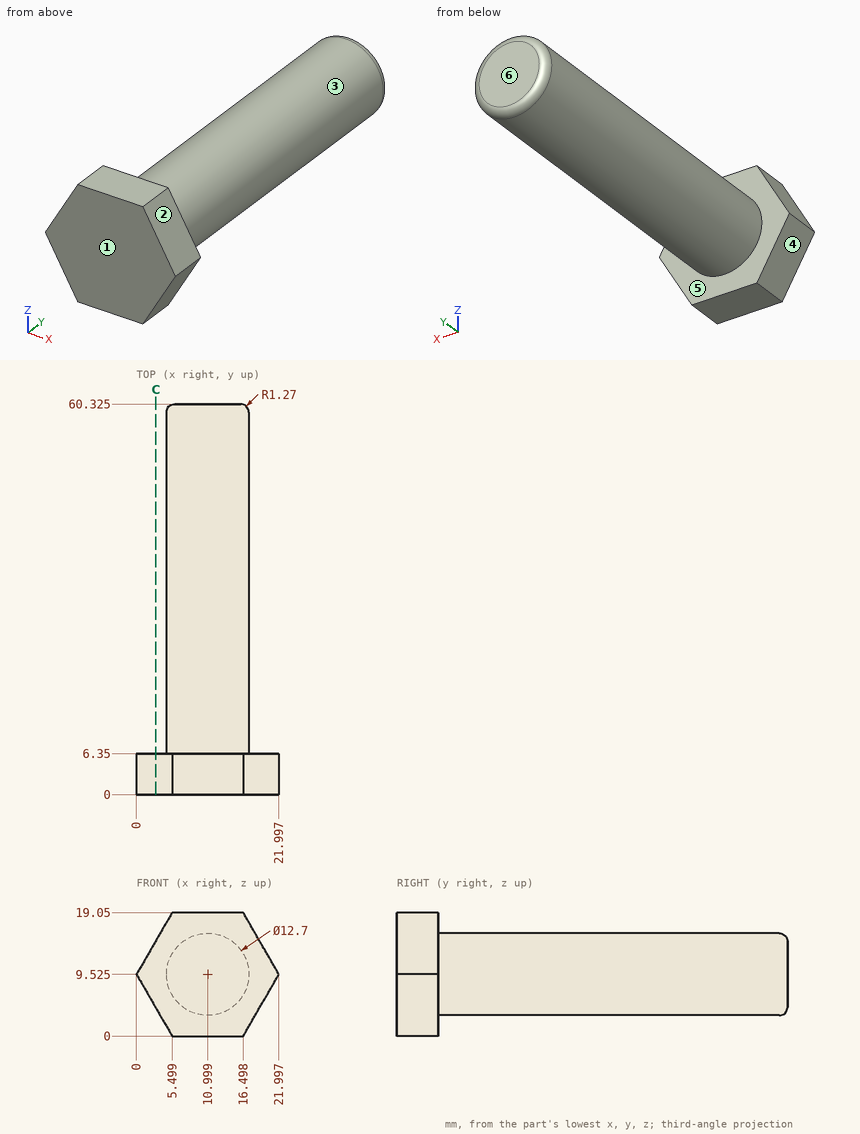
Here's the drawing with two shaded views (mm, measured from the low corner). I have some questions. A direction names the side the tool comes from. Coordinates: 2 decimals unless noted, no trailing zeros. Loops run counter-clockwise (first coordinate to the right, second up) from the corner with the lowest first, then second, coordinate; pieces in that order, holes last. Notation, with made-up numbers: (-26.5, 72) -> (12.5, 72) arc R6 ccw to (12.5, 76) -> close; hole circle Ø11 at (14, 62). An arc over 180 degrees is marked (long way). Use one line per item in the form item = value. Start each with the question number.
(1) Will these pins go through, and if not, where does the flat tip stop? pin 1 (1.5 mm diameter, centred on y = 46, z = 7, fed in from -X); pin 2 (10 mm diameter, centred on x = 16.5, z = 17, fed in from -Y); pin 3 (5 mm diameter, centred on y = 42.5, z = 9.5, fed in from +X); pin 4 (3 mm diameter, centred on y = 17, z = 7, fed in from -X).
(2) If we section it at C-C (x = 3): Please give me the cut outline in (y, z).
(3) On a 3-axis mill with a long thin cutter (end or side, diameter ignored), from which of +Z, -Z, +X, -X, +Y, -Y can I reach the whole of each face in a straight line? I mean the marked faces 5 and 6. Say none if no direction works.
(4) Please list where these lines run through material, in increasing order: line 1 along Y through (x, z) = (3.75, 13.75); line 2 along Y through (x, z) = (15.75, 7.25); line 3 along Z through (x, y) = (10, 39) (1 decimal).
(5) We'd pull the mould along X, two halves only. Please class the marked faces 1, 2, 3 and 4: pulls with the +X half, pulls with the -X half, needs draft (parallel to the pull), parting line crosses it, or undercut.
Verdict:
q1.pin_1 = 4.9
q1.pin_2 = 0
q1.pin_3 = 17.35
q1.pin_4 = 4.73
q2.outline = (0, 4.33) -> (6.35, 4.33) -> (6.35, 14.72) -> (0, 14.72) -> close
q3.face_5 = +Y
q3.face_6 = +Z, -Z, +X, -X, +Y
q4.line_1 = 0 to 6.35
q4.line_2 = 0 to 60.31
q4.line_3 = 3.3 to 15.8
q5.face_1 = needs draft
q5.face_2 = pulls with the +X half
q5.face_3 = parting line crosses it
q5.face_4 = pulls with the -X half
